Geometry check sheet. Reference: the model listing, model coordinates, mm. Face numbers are marked on the shaded views. Coordinates: 2 decimals unless noted, no trailing zeros. Use CSV: the item, a comma, the result in double quotes.
```python
from build123d import *

# Parameters (mm, degrees)
F1_DEPTH = 9.525
F3_DEPTH = 6.35
F4_R     = 1.5875
F5_R     = 1.5875


with BuildPart() as f1:
    # F0 (on Top) → F1 (new body)
    with BuildSketch(Plane.XY):
        with BuildLine():
            ThreePointArc((0, 6.35), (1.8598719395, 1.8598719395), (6.35, 0))
            Line((6.35, 0), (95.25, 0))
            ThreePointArc((95.25, 0), (99.7401280605, 1.8598719395), (101.6, 6.35))
            Line((101.6, 6.35), (101.6, 69.85))
            ThreePointArc((101.6, 69.85), (99.7401280605, 74.3401280605), (95.25, 76.2))
            Line((95.25, 76.2), (6.35, 76.2))
            ThreePointArc((6.35, 76.2), (1.8598719395, 74.3401280605), (0, 69.85))
            Line((0, 69.85), (0, 6.35))
        make_face()
    extrude(amount=F1_DEPTH)

    # F2 (on face) → F3 (cut)
    with BuildSketch(Plane.XY.offset(9.525)):
        with BuildLine():
            ThreePointArc((96.8375, 65.0875), (94.9776280605, 69.5776280605), (90.4875, 71.4375))
            Line((90.4875, 71.4375), (11.1125, 71.4375))
            ThreePointArc((11.1125, 71.4375), (6.6223719395, 69.5776280605), (4.7625, 65.0875))
            Line((4.7625, 65.0875), (4.7625, 11.1125))
            ThreePointArc((4.7625, 11.1125), (6.6223719395, 6.6223719395), (11.1125, 4.7625))
            Line((11.1125, 4.7625), (90.4875, 4.7625))
            ThreePointArc((90.4875, 4.7625), (94.9776280605, 6.6223719395), (96.8375, 11.1125))
            Line((96.8375, 11.1125), (96.8375, 65.0875))
        make_face()
    extrude(amount=-F3_DEPTH, mode=Mode.SUBTRACT)

    # F4
    f4_edges = [f1.edges().sort_by_distance(p)[0] for p in [
        (0, 38.1, 9.525),
        (1.859872, 74.340128, 9.525),
        (1.859872, 1.859872, 9.525),
        (50.8, 76.2, 9.525),
        (50.8, 0, 9.525),
        (99.740128, 74.340128, 9.525),
        (99.740128, 1.859872, 9.525),
        (101.6, 38.1, 9.525),
        (94.977628, 6.622372, 9.525),
        (96.8375, 38.1, 9.525),
        (94.977628, 69.577628, 9.525),
        (50.8, 71.4375, 9.525),
        (6.622372, 69.577628, 9.525),
        (4.7625, 38.1, 9.525),
        (6.622372, 6.622372, 9.525),
        (50.8, 4.7625, 9.525),
        (0, 38.1, 0),
        (1.859872, 1.859872, 0),
        (50.8, 0, 0),
        (99.740128, 1.859872, 0),
        (101.6, 38.1, 0),
        (99.740128, 74.340128, 0),
        (50.8, 76.2, 0),
        (1.859872, 74.340128, 0),
    ]]
    fillet(f4_edges, radius=F4_R)

    # F5
    f5_edges = [f1.edges().sort_by_distance(p)[0] for p in [
        (94.977628, 6.622372, 3.175),
        (96.8375, 38.1, 3.175),
        (94.977628, 69.577628, 3.175),
        (50.8, 71.4375, 3.175),
        (6.622372, 69.577628, 3.175),
        (4.7625, 38.1, 3.175),
        (6.622372, 6.622372, 3.175),
        (50.8, 4.7625, 3.175),
    ]]
    fillet(f5_edges, radius=F5_R)


solid = f1.part
```
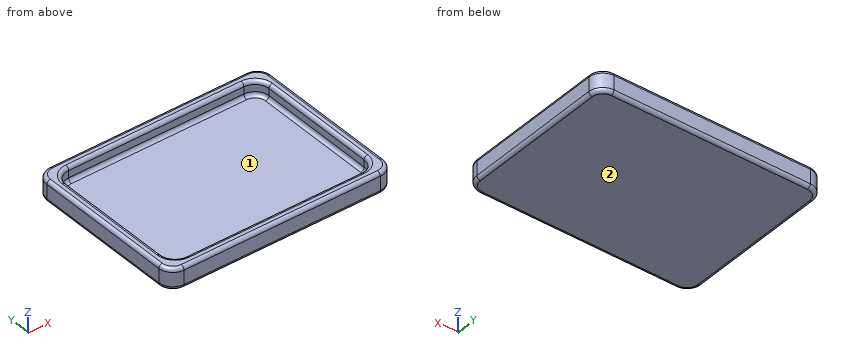
1. Thickness scan on line 1 (X direction, y = 55.5, z = 7.75); line 2 (Y direction, x = 79, z = 4.5); line 3 (Z direction, x = 92, y = 29) (3 decimals). Record the ranges inside material, lowest first. Write a range as [from, to].
The answers:
line 1,"[0, 4.76], [96.84, 101.6]"
line 2,"[0, 4.78], [71.42, 76.2]"
line 3,"[0, 3.175]"
2. Release check for a two-part mould opening along Y. For the marked faces 1 and 2 record: +Y half, -Y half, draft (parallel to the pull), parting line (faces both ways), or undercut.
The answers:
face 1,"undercut"
face 2,"draft"
3. Gauge pin test, flat end, axial feed: P1, Ø19, axis at x = 31, y = 41, coming from the +Z side (3 decimals). Record the tip position at first contact, or that the pin passes through.
The answers:
P1,"z = 3.175"
